The model under review builds one solid part; all positions refer to its coordinate system, in mm. A direction names the side the tool comes from. Give positions to 0.01 mm unless a question says otherwise; leave off trailing zeros. Order: outer loops, then holes, each group sorted by start corner. A loop starts at its lowest first (then second) coordinate and runs counter-clockwise, first axis right, second up. Notation, with made-up numbers: M 11.5,7 L 49.5,7 A30 cw 49.5,41 Z; hole C 25.25,55 d3. An arc over 180 degrees is marked long. One line per question, with ' | ' between items. Start each with the question number.
1. Wall thickness on L1, parallel to Y at x = 143, z = -0.3; L2, parallel to X at y = 246, z = -0.75; L3, parallel to X at y = 459, z = -1.3: over which ranges is each line inside the solid? List them lowest first.
2. For faces 1 (the face through (125, 457, -1)), 2 (the face through (163, 244, 0)), list the 3-axis set-ups (+Z, -Z, +X, -X, +Y, -Y) from which the entire face can be reached by the end or side of a thin tool; tool diameter is ignored.
3. Insertion check: P1, Ø4.5, axis at x = 164.74, y = 348.08, coming from the -Z side. The pin has a flat end and moves straight along its axis. Give the tip position at first contact, or say it passes through.
4. We need section A-A on x = 147. Write out the cut boundary in (y, z), then the cut area to 3 significant figures.
```python
from build123d import *

# Parameters (mm, degrees)
CONVERT_SOLID1_START     = -1.5
CONVERT_SOLID1_OUTLINE_R = 2
CONVERT_SOLID1_DEPTH     = 1.5


# Read off the part's stored shape, not the designer's step: Convert-Solid1
with BuildPart() as part:
    # Convert-Solid1 outline → Convert-Solid1 (new body)
    with BuildSketch(Plane.XY.offset(CONVERT_SOLID1_START)):
        with BuildLine():
            Line((330, 2), (330, 480))
            ThreePointArc((330, 480), (329.414213562, 481.414213562), (328, 482))
            Line((328, 482), (2, 482))
            ThreePointArc((2, 482), (0.585786438, 481.414213562), (0, 480))
            Line((0, 480), (0, 2))
            ThreePointArc((0, 2), (0.585786438, 0.585786438), (2, 0))
            Line((2, 0), (328, 0))
            ThreePointArc((328, 0), (329.414213562, 0.585786438), (330, 2))
        make_face()
        with BuildLine():
            ThreePointArc((23.25, 23.65), (24.9, 22), (23.25, 20.35))
            Line((23.25, 20.35), (22.25, 20.35))
            ThreePointArc((22.25, 20.35), (20.6, 22), (22.25, 23.65))
            Line((22.25, 23.65), (23.25, 23.65))
        make_face(mode=Mode.SUBTRACT)
        with BuildLine():
            ThreePointArc((23.25, 98.65), (24.9, 97), (23.25, 95.35))
            Line((23.25, 95.35), (22.25, 95.35))
            ThreePointArc((22.25, 95.35), (20.6, 97), (22.25, 98.65))
            Line((22.25, 98.65), (23.25, 98.65))
        make_face(mode=Mode.SUBTRACT)
        with BuildLine():
            ThreePointArc((23.25, 173.65), (24.9, 172), (23.25, 170.35))
            Line((23.25, 170.35), (22.25, 170.35))
            ThreePointArc((22.25, 170.35), (20.6, 172), (22.25, 173.65))
            Line((22.25, 173.65), (23.25, 173.65))
        make_face(mode=Mode.SUBTRACT)
        with BuildLine():
            ThreePointArc((307.75, 23.65), (309.4, 22), (307.75, 20.35))
            Line((307.75, 20.35), (306.75, 20.35))
            ThreePointArc((306.75, 20.35), (305.1, 22), (306.75, 23.65))
            Line((306.75, 23.65), (307.75, 23.65))
        make_face(mode=Mode.SUBTRACT)
        with BuildLine():
            ThreePointArc((307.75, 98.65), (309.4, 97), (307.75, 95.35))
            Line((307.75, 95.35), (306.75, 95.35))
            ThreePointArc((306.75, 95.35), (305.1, 97), (306.75, 98.65))
            Line((306.75, 98.65), (307.75, 98.65))
        make_face(mode=Mode.SUBTRACT)
        with BuildLine():
            ThreePointArc((307.75, 173.65), (309.4, 172), (307.75, 170.35))
            Line((307.75, 170.35), (306.75, 170.35))
            ThreePointArc((306.75, 170.35), (305.1, 172), (306.75, 173.65))
            Line((306.75, 173.65), (307.75, 173.65))
        make_face(mode=Mode.SUBTRACT)
        with BuildLine():
            ThreePointArc((23.25, 248.65), (24.9, 247), (23.25, 245.35))
            Line((23.25, 245.35), (22.25, 245.35))
            ThreePointArc((22.25, 245.35), (20.6, 247), (22.25, 248.65))
            Line((22.25, 248.65), (23.25, 248.65))
        make_face(mode=Mode.SUBTRACT)
        with BuildLine():
            ThreePointArc((23.25, 323.65), (24.9, 322), (23.25, 320.35))
            Line((23.25, 320.35), (22.25, 320.35))
            ThreePointArc((22.25, 320.35), (20.6, 322), (22.25, 323.65))
            Line((22.25, 323.65), (23.25, 323.65))
        make_face(mode=Mode.SUBTRACT)
        with BuildLine():
            ThreePointArc((8.23683607, 345.178083895), (10.33683607, 343.078083895), (8.23683607, 340.978083895))
            Line((8.23683607, 340.978083895), (7.23683607, 340.978083895))
            ThreePointArc((7.23683607, 340.978083895), (5.13683607, 343.078083895), (7.23683607, 345.178083895))
            Line((7.23683607, 345.178083895), (8.23683607, 345.178083895))
        make_face(mode=Mode.SUBTRACT)
        with Locations((164.73683607, 348.078083895)):
            Circle(CONVERT_SOLID1_OUTLINE_R, mode=Mode.SUBTRACT)
        with BuildLine():
            ThreePointArc((6.73683607, 372.678083895), (8.83683607, 370.578083895), (6.73683607, 368.478083895))
            Line((6.73683607, 368.478083895), (5.73683607, 368.478083895))
            ThreePointArc((5.73683607, 368.478083895), (3.63683607, 370.578083895), (5.73683607, 372.678083895))
            Line((5.73683607, 372.678083895), (6.73683607, 372.678083895))
        make_face(mode=Mode.SUBTRACT)
        with BuildLine():
            ThreePointArc((23.25, 398.65), (24.9, 397), (23.25, 395.35))
            Line((23.25, 395.35), (22.25, 395.35))
            ThreePointArc((22.25, 395.35), (20.6, 397), (22.25, 398.65))
            Line((22.25, 398.65), (23.25, 398.65))
        make_face(mode=Mode.SUBTRACT)
        with BuildLine():
            ThreePointArc((23.25, 473.65), (24.9, 472), (23.25, 470.35))
            Line((23.25, 470.35), (22.25, 470.35))
            ThreePointArc((22.25, 470.35), (20.6, 472), (22.25, 473.65))
            Line((22.25, 473.65), (23.25, 473.65))
        make_face(mode=Mode.SUBTRACT)
        with BuildLine():
            ThreePointArc((118.083333333, 443.65), (119.733333333, 442), (118.083333333, 440.35))
            Line((118.083333333, 440.35), (117.083333333, 440.35))
            ThreePointArc((117.083333333, 440.35), (115.433333333, 442), (117.083333333, 443.65))
            Line((117.083333333, 443.65), (118.083333333, 443.65))
        make_face(mode=Mode.SUBTRACT)
        with BuildLine():
            ThreePointArc((118.083333333, 473.65), (119.733333333, 472), (118.083333333, 470.35))
            Line((118.083333333, 470.35), (117.083333333, 470.35))
            ThreePointArc((117.083333333, 470.35), (115.433333333, 472), (117.083333333, 473.65))
            Line((117.083333333, 473.65), (118.083333333, 473.65))
        make_face(mode=Mode.SUBTRACT)
        with Locations((216.13683607, 348.078083895)):
            Circle(CONVERT_SOLID1_OUTLINE_R, mode=Mode.SUBTRACT)
        with BuildLine():
            ThreePointArc((307.75, 248.65), (309.4, 247), (307.75, 245.35))
            Line((307.75, 245.35), (306.75, 245.35))
            ThreePointArc((306.75, 245.35), (305.1, 247), (306.75, 248.65))
            Line((306.75, 248.65), (307.75, 248.65))
        make_face(mode=Mode.SUBTRACT)
        with BuildLine():
            ThreePointArc((307.75, 323.65), (309.4, 322), (307.75, 320.35))
            Line((307.75, 320.35), (306.75, 320.35))
            ThreePointArc((306.75, 320.35), (305.1, 322), (306.75, 323.65))
            Line((306.75, 323.65), (307.75, 323.65))
        make_face(mode=Mode.SUBTRACT)
        with BuildLine():
            ThreePointArc((322.76316393, 345.178083895), (324.86316393, 343.078083895), (322.76316393, 340.978083895))
            Line((322.76316393, 340.978083895), (321.76316393, 340.978083895))
            ThreePointArc((321.76316393, 340.978083895), (319.66316393, 343.078083895), (321.76316393, 345.178083895))
            Line((321.76316393, 345.178083895), (322.76316393, 345.178083895))
        make_face(mode=Mode.SUBTRACT)
        with BuildLine():
            ThreePointArc((195, 467), (205, 457), (195, 447))
            Line((195, 447), (135, 447))
            ThreePointArc((135, 447), (125, 457), (135, 467))
            Line((135, 467), (195, 467))
        make_face(mode=Mode.SUBTRACT)
        with BuildLine():
            ThreePointArc((212.916666667, 443.65), (214.566666667, 442), (212.916666667, 440.35))
            Line((212.916666667, 440.35), (211.916666667, 440.35))
            ThreePointArc((211.916666667, 440.35), (210.266666667, 442), (211.916666667, 443.65))
            Line((211.916666667, 443.65), (212.916666667, 443.65))
        make_face(mode=Mode.SUBTRACT)
        with BuildLine():
            ThreePointArc((212.916666667, 473.65), (214.566666667, 472), (212.916666667, 470.35))
            Line((212.916666667, 470.35), (211.916666667, 470.35))
            ThreePointArc((211.916666667, 470.35), (210.266666667, 472), (211.916666667, 473.65))
            Line((211.916666667, 473.65), (212.916666667, 473.65))
        make_face(mode=Mode.SUBTRACT)
        with BuildLine():
            ThreePointArc((324.26316393, 372.678083895), (326.36316393, 370.578083895), (324.26316393, 368.478083895))
            Line((324.26316393, 368.478083895), (323.26316393, 368.478083895))
            ThreePointArc((323.26316393, 368.478083895), (321.16316393, 370.578083895), (323.26316393, 372.678083895))
            Line((323.26316393, 372.678083895), (324.26316393, 372.678083895))
        make_face(mode=Mode.SUBTRACT)
        with BuildLine():
            ThreePointArc((307.75, 398.65), (309.4, 397), (307.75, 395.35))
            Line((307.75, 395.35), (306.75, 395.35))
            ThreePointArc((306.75, 395.35), (305.1, 397), (306.75, 398.65))
            Line((306.75, 398.65), (307.75, 398.65))
        make_face(mode=Mode.SUBTRACT)
        with BuildLine():
            ThreePointArc((307.75, 473.65), (309.4, 472), (307.75, 470.35))
            Line((307.75, 470.35), (306.75, 470.35))
            ThreePointArc((306.75, 470.35), (305.1, 472), (306.75, 473.65))
            Line((306.75, 473.65), (307.75, 473.65))
        make_face(mode=Mode.SUBTRACT)
    extrude(amount=CONVERT_SOLID1_DEPTH)


solid = part.part
```
Entries:
1) L1: y = 0 to 447, 467 to 482 | L2: x = 0 to 20.94, 24.56 to 305.44, 309.06 to 330 | L3: x = 0 to 125.2, 204.8 to 330
2) face 1: +Z, -Z | face 2: +Z, +X, -X, +Y, -Y
3) P1: stops at z = -1.5
4) outline: M 0,-1.5 L 447,-1.5 L 447,0 L 0,0 Z; M 467,-1.5 L 482,-1.5 L 482,0 L 467,0 Z | area: 693 mm^2
